Job drawing, mm, ordinate dimensions from the low corner. One solid piece. A direction names the side the tool comes from. Round coordinates to 2 decimals unless told otherwise and drop trailing zeros. Loops run counter-clockwise (first coordinate to the right, second up) from the corner with the lowest first, then second, coordinate; pieces in that order, holes last. Notation, with made-up numbers: M 68.5,58 L 127.5,58 A15 ccw 127.5,73 Z; hole C 21,-3 d6. An arc over 180 degrees is marked long. Put each result on its own line as item: value. Start each with the question number.
1) Which spindle directions (+Z, -Z, +X, -X, +Y, -Y) get a long thin tool onto all of the face, cutting with end or side? Do the marked faces 1 and 2. Say none if no direction does.
2) Slice it at D-D on x = 20. Give the cut face in (y, z), then the cut area to 3 significant figures.
3) Slice it at A-A on x = 16. Give the cut face in (y, z).
4) Slice it at B-B on y = 2. Give the cut face in (x, z), then the cut area to 3 significant figures.
5) Slice it at C-C on z = 19. Give the cut face in (x, y), then the cut area to 3 significant figures.
6) Probe line 1 along X through (y, z) = (2.35, 25); line 2 along Z through (x, y) = (20, 3.4); line 3 along Y through (x, z) = (28.5, 10). List the from-to ranges inside material, lowest first.
7) Drop flat-ended pins along their axis: pin 1 Ø2 at (y, z) = (24, 45) entering from +X; pin 2 Ø15 at (x, z) = (15, 29) entering from +Y. Give the stop position or say it passes through.
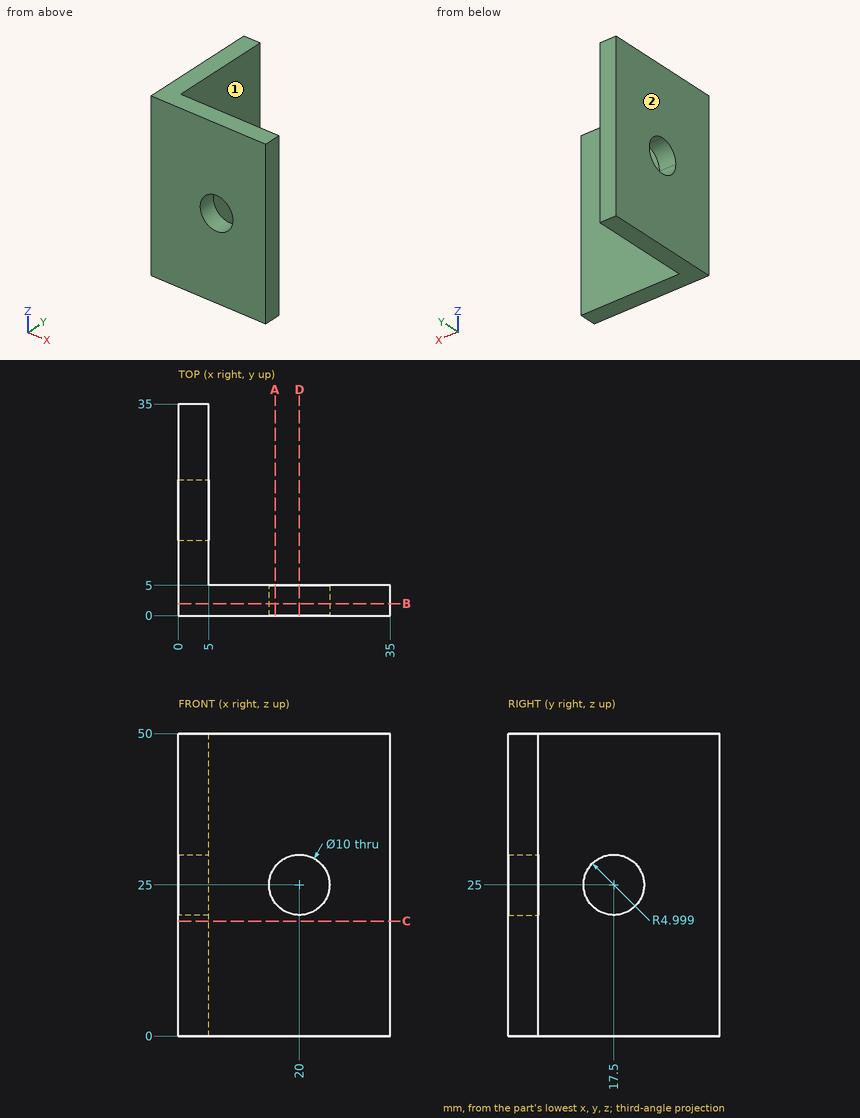
Recorded:
1. face 1: +Z, -Z, +X, +Y
1. face 2: +Z, -Z, -X, +Y, -Y
2. outline: M 0,0 L 5,0 L 5,20 L 0,20 Z; M 0,30 L 5,30 L 5,50 L 0,50 Z
2. area: 200 mm2
3. outline: M 0,0 L 5,0 L 5,22 L 0,22 Z; M 0,28 L 5,28 L 5,50 L 0,50 Z
4. outline: M 0,0 L 35,0 L 35,50 L 0,50 Z; hole C 20,25 d10
4. area: 1,670 mm2
5. outline: M 0,0 L 35,0 L 35,5 L 5,5 L 5,35 L 0,35 Z
5. area: 325 mm2
6. line 1: x = 0 to 15, 25 to 35
6. line 2: z = 0 to 20, 30 to 50
6. line 3: y = 0 to 5
7. pin 1: stops at x = 5
7. pin 2: stops at y = 5
